from build123d import *

# Parameters (mm, degrees)
ESQUISSE1_R                  = 2
BOSS_EXTRU_1_DEPTH           = 24
ENL_V_MAT_EXTRU_1_DEPTH      = 24
ENL_V_MAT_EXTRU_1_DEPTH_BACK = 24
ESQUISSE2_R                  = 2
ESQUISSE2_W                  = 6
ESQUISSE2_H                  = 11.5
CHANFREIN1_SIZE              = 1.5


with BuildPart() as part:
    # Esquisse1 → Boss.-Extru.1 (new body)
    with BuildSketch(Plane(origin=(0, 0, 0), x_dir=(0, 0, -1), z_dir=(1, 0, 0))):
        with BuildLine():
            Line((-8.240740741, 1.277777778), (1.259259259, 1.277777778))
            Line((1.259259259, 1.277777778), (1.259259259, 5.277777778))
            ThreePointArc((1.259259259, 5.277777778), (1.845045697, 6.69199134), (3.259259259, 7.277777778))
            Line((3.259259259, 7.277777778), (7.259259259, 7.277777778))
            ThreePointArc((7.259259259, 7.277777778), (8.673472822, 6.69199134), (9.259259259, 5.277777778))
            Line((9.259259259, 5.277777778), (9.259259259, 0.277777778))
            ThreePointArc((9.259259259, 0.277777778), (8.673472822, -1.136435785), (7.259259259, -1.722222222))
            Line((7.259259259, -1.722222222), (-8.240740741, -1.722222222))
            Line((-8.240740741, -1.722222222), (-8.240740741, 1.277777778))
        make_face()
        with Locations((5.259259259, 3.401253161)):
            Circle(ESQUISSE1_R, mode=Mode.SUBTRACT)
    extrude(amount=BOSS_EXTRU_1_DEPTH)

    # Esquisse2 → Enlèv. mat.-Extru.1 (cut, two sides: drawn at the far end of the back side and taken through both)
    with BuildSketch(Plane(origin=(0, 1.277777778, 0), x_dir=(1, 0, 0), z_dir=(0, 1, 0)).offset(-ENL_V_MAT_EXTRU_1_DEPTH_BACK)):
        with Locations(Location((19, -3.490740741, 0), (0, 0, 90))):
            Circle(ESQUISSE2_R)
        with Locations(Location((5, -3.490740741, 0), (0, 0, 90))):
            Circle(ESQUISSE2_R)
        with Locations((12, 3.509259259)):
            Rectangle(ESQUISSE2_W, ESQUISSE2_H)
    extrude(amount=ENL_V_MAT_EXTRU_1_DEPTH + ENL_V_MAT_EXTRU_1_DEPTH_BACK, mode=Mode.SUBTRACT)

    # Chanfrein1
    chanfrein1_edges = [part.edges().sort_by_distance(p)[0] for p in [
        (24, 3.401253161, -3.259259259),
        (19, 1.277777778, 5.490740741),
        (5, 1.277777778, 5.490740741),
    ]]
    chamfer(chanfrein1_edges, length=CHANFREIN1_SIZE)


solid = part.part
Input: part model. Units: mm. Frame: model coordinates. A direction names the side the tool comes from. Give positions to 0.01 mm unless a question says otherwise; leave off trailing zeros. Order: outer loops, then holes, each group sorted by start corner. A loop starts at its lowest first (then second) coordinate and runs counter-clockwise, first axis right, second up. Notation, with made-up numbers: (-28.5, 25.5) - (3.5, 25.5) arc R15 cw to (3.5, 52.5) - close; hole circle Ø11 at (54, 74). An arc over 180 degrees is marked (long way). Answer as a JSON object with one key per item and string values. Group by question number.
Q1. Line query: probe 1 along X at (y, z) = (0.5, 0); probe 2 along X at (y, z) = (1, 2.5); probe 3 along X at (y, z) = (0, 1.5). Output: solid intervals per line, ascending.
Q2. Cut plane C-C, the plane x = 13.25. Output: boundary loops of the cut face in (y, z).
Q3. Cut plane B-B, the plane y = -0.5. Output: boundary loops of the cut face in (x, z), then the cut area to 3 significant figures.
Q4. Set-up query: faces 5 (the face through (7.1, -0.1, 3.8)), 6 (the face through (19, 3, -1.259)), 7 (the face through (9, 2, -3)). Return all of +Z, -Z, +X, -X, +Y, -Y with unobstructed straight access to the full face (end or side cutting, diameter ignored); none if empty.
Q5. First-contact query: pin 1 Ø1.5 at (x, y) = (11.5, -0.5) entering from -Z; pin 2 Ø2 at (x, y) = (18.5, 3) entering from +Z; pin 3 Ø3.5 at (y, z) = (3.4, -5.26) entering from -X; pin 4 Ø6.5 at (x, z) = (5, 3.49) entering from +Y. Flat tips, straight axial feed; report the tip coordinate or a pass-through.
Q6. Cut plane A-A, the plane x = 19. Output: boundary loops of the cut face in (y, z).
Q7. Mould query, pull axis X, two halves, no side actions, for faces 1 (the face through (0, 2, -3)), 2 (the face through (12, 0, 2.241)), 3 (the face through (24, 1, -1)), 4 (the face through (4, 3, -9.259)). Classes: pulls with the +X half, pulls with the -X half, needs draft (parallel to the pull), parting line crosses it, or undercut.
Results:
{
 "1": {"probe 1": "0 to 9, 15 to 24", "probe 2": "0 to 1.93, 8.07 to 15.93, 22.07 to 24", "probe 3": "0 to 4.01, 5.99 to 9, 15 to 18.01, 19.99 to 24"},
 "2": {"outline": "(-1.72, 2.24) - (1.28, 2.24) - (1.28, 8.24) - (-1.72, 8.24) - close"},
 "3": {"outline": "(0, -9.1) - (9, -9.1) - (9, 2.24) - (15, 2.24) - (15, -9.1) - (24, -9.1) - (24, 8.24) - (0, 8.24) - close; hole circle Ø4 at (5, 3.49); hole circle Ø4 at (19, 3.49)", "area": "323 mm^2"},
 "4": {"face 5": "+Y", "face 6": "+Z, +X, -X, +Y", "face 7": "-Z, +Y, -Y"},
 "5": {"pin 1": "z = 2.24", "pin 2": "z = -1.26", "pin 3": "through", "pin 4": "y = 1.03"},
 "6": {"outline": "(-1.72, -7.26) arc R2 ccw to (0.28, -9.26) - (5.28, -9.26) arc R2 ccw to (7.28, -7.26) - (7.28, -3.26) arc R2 ccw to (5.28, -1.26) - (1.28, -1.26) - (1.28, -0.01) - (-0.22, 1.49) - (-1.72, 1.49) - close; (-1.72, 5.49) - (-0.22, 5.49) - (1.28, 6.99) - (1.28, 8.24) - (-1.72, 8.24) - close; hole circle Ø4 at (3.4, -5.26)"},
 "7": {"face 1": "pulls with the -X half", "face 2": "undercut", "face 3": "pulls with the +X half", "face 4": "needs draft"}
}
